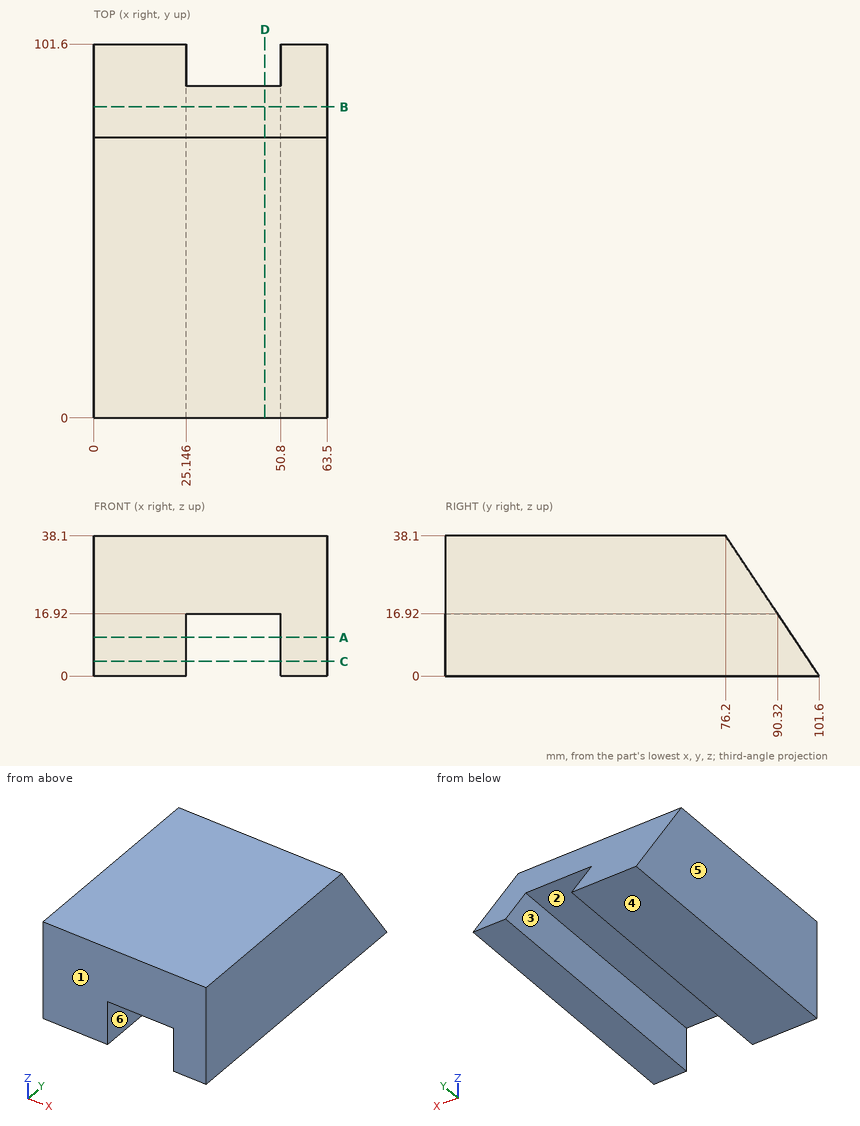
Geometry: see drawing. Coordinates: mm, zero at the bounding-box minimum. A direction names the side the tool comes from. Give positions to 0.01 mm unless a question says otherwise; leave off trailing zeros. Loops run counter-clockwise (first coordinate to the right, second up) from the corner with the lowest first, then second, coordinate; pieces in that order, holes last. Notation, with made-up numbers: (-0.75, -8) - (12.25, -8) arc R16 ccw to (12.25, 5) - close; hole circle Ø11 at (45.5, -22). An arc over 180 degrees is marked (long way). Answer as CSV lines item,"result". Start each with the question number.
1. Ray query, L1, parallel to X at y = 52, z = 7; L2, parallel to Z at x = 42, y = 31; L3, parallel to Y at x = 4, z = 10.5. Return the intervals inside material, ascending.
2. Section C-C, the plane z = 4. Return loops of the section in (x, y), plus the area to 3 significant figures.
3. Draft query along X for the marked faces 3, 4, 5 and 6. Return one class per face: released by +X, released by -X, zero draft, split by the parting line, or undercut.
4. Section D-D, the plane x = 46.5. Return loops of the section in (y, z), plus the area to 3 significant figures.
5. Section B-B, the plane y = 84.5. Return loops of the section in (x, z).
6. Section A-A, the plane z = 10.5. Return loops of the section in (x, y), plus the area to 3 significant figures.
7. Pin query (flat end, axial travel): P1, Ø10, axis at y = 49.5, z = 7, coming from the -X side; P2, Ø6, axis at x = 11.5, z = 25.5, coming from the +Y side; P3, Ø3, axis at x = 53, z = 33, coming from the +Y side; P4, Ø6, axis at x = 24, z = 27.5, coming from the +Y side. Return the tip coordinate at first contact, or that it passes through.
8. Reachability of the marked faces 1 and 2 from +Z, -Z, +X, -X, +Y, -Y: full face, straight path, thin tool, end or side. Return the list, or none.
Answers:
1,L1,"x = 0 to 25.15, 50.8 to 63.5"
1,L2,"z = 16.92 to 38.1"
1,L3,"y = 0 to 94.6"
2,outline,"(0, 0) - (25.15, 0) - (25.15, 98.93) - (0, 98.93) - close; (50.8, 0) - (63.5, 0) - (63.5, 98.93) - (50.8, 98.93) - close"
2,area,"3,740 mm2"
3,face 3,"undercut"
3,face 4,"zero draft"
3,face 5,"released by -X"
3,face 6,"undercut"
4,outline,"(0, 16.92) - (90.32, 16.92) - (76.2, 38.1) - (0, 38.1) - close"
4,area,"1,760 mm2"
5,outline,"(0, 0) - (25.15, 0) - (25.15, 16.92) - (50.8, 16.92) - (50.8, 0) - (63.5, 0) - (63.5, 25.65) - (0, 25.65) - close"
6,outline,"(0, 0) - (25.15, 0) - (25.15, 94.6) - (0, 94.6) - close; (50.8, 0) - (63.5, 0) - (63.5, 94.6) - (50.8, 94.6) - close"
6,area,"3,580 mm2"
7,P1,"stops at x = 0"
7,P2,"stops at y = 86.6"
7,P3,"stops at y = 80.6"
7,P4,"stops at y = 85.27"
8,face 1,"+Z, -Z, +X, -X, -Y"
8,face 2,"-Z, +Y, -Y"
